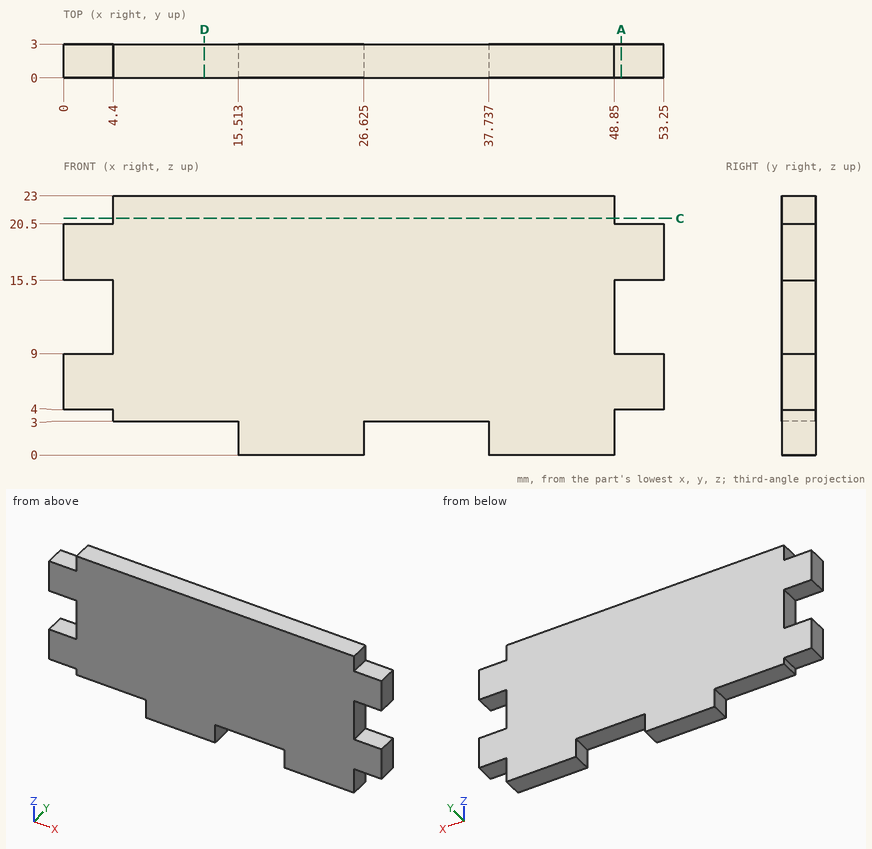
Drawing for the job (mm, zero at the part's lowest x, y, z). Give positions to 0.01 mm unless a question says otherwise; leave off trailing zeros. Order: outer loops, then holes, each group sorted by start corner. A loop starts at its lowest first (then second) coordinate and runs counter-clockwise, first axis right, second up. Notation, with made-up numbers: M 21.25,62.5 L 73.25,62.5 A5 cw 73.25,71.5 Z; hole C 67.25,61 d7. An arc over 180 degrees is marked long. Put each result on its own line as item: value.
Item 1: Slice it at D-D, the plane x = 12.5. Write the cut outline in (y, z).
From the geometry:
outline: M 0,3 L 3,3 L 3,23 L 0,23 Z
Item 2: Slice it at A-A, the plane x = 49.5. Write the cut outline in (y, z).
From the geometry:
outline: M 0,4 L 3,4 L 3,9 L 0,9 Z; M 0,15.5 L 3,15.5 L 3,20.5 L 0,20.5 Z
Item 3: Probe line 1 (Z direction, x = 30, y = 1); line 2 (X direction, y = 1.7, z = 11.25). List the from-to ranges inside material, lowest first. Write a range as [from, to].
From the geometry:
line 1: z = [3, 23]
line 2: x = [4.4, 48.85]
Item 4: Slice it at C-C, the plane z = 21. Write the cut outline in (x, y), plus the area to 3 significant figures.
From the geometry:
outline: M 4.4,0 L 48.85,0 L 48.85,3 L 4.4,3 Z
area: 133 mm2
Item 5: Flat gauge pins, fed straight in: pin 1 Ø0.9 at (x, y) = (2, 1.5) entering from +Z; pin 2 Ø1.5 at (y, z) = (2, 2) entering from -X; pin 3 Ø1.5 at (x, y) = (50, 2) entering from -Z. Where does each tip first touch, or does it go through?
From the geometry:
pin 1: stops at z = 20.5
pin 2: stops at x = 15.51
pin 3: stops at z = 4
